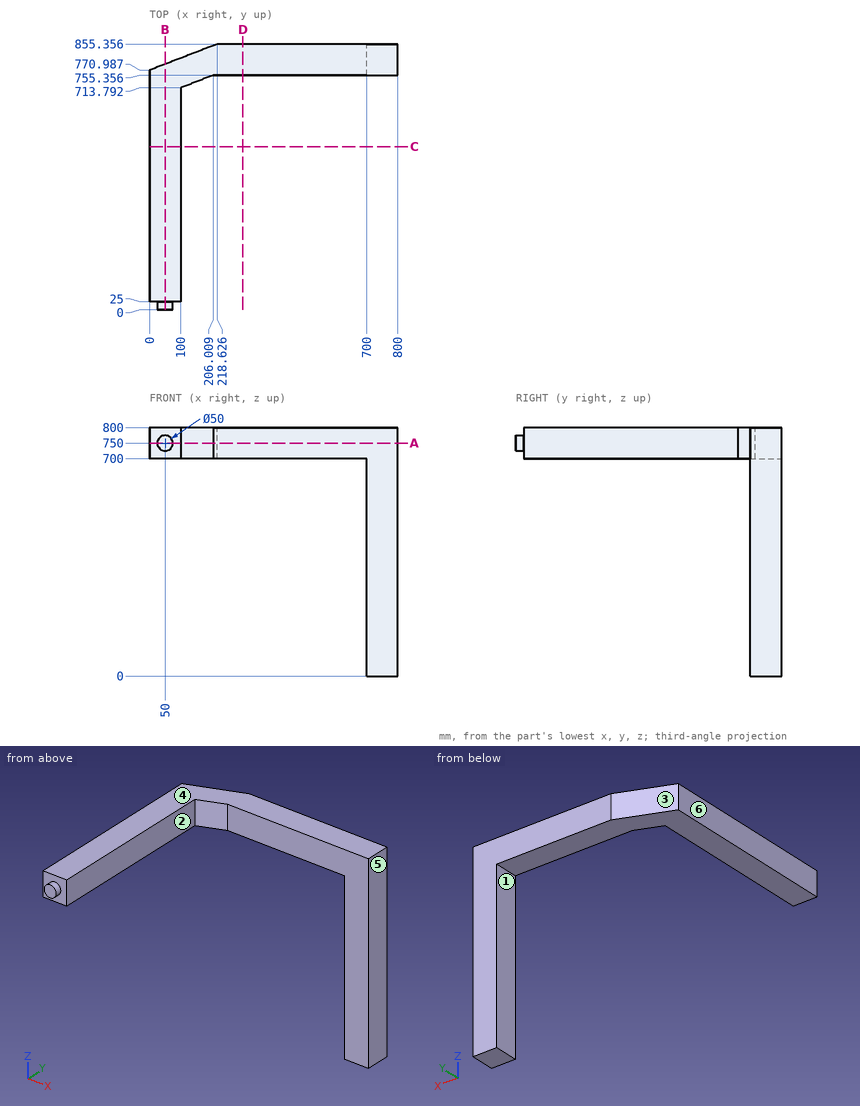
The drawing under review shows one solid part. Ordinate dimensions are in mm from its lowest x, y, z. A direction names the side the tool comes from. Round coordinates to 2 decimals unless told otherwise and drop trailing zeros. Order: outer loops, then holes, each group sorted by start corner. A loop starts at its lowest first (then second) coordinate and runs counter-clockwise, first axis right, second up. Notation, with made-up numbers: (8, 83.5) -> (28, 83.5) arc R12 cw to (28, 94.5) -> close; hole circle Ø9 at (64.25, 39.25). An arc over 180 degrees is marked (long way). Use a Markdown table: item, result.
Q1. We need section A-A on z = 750. Write out the cut boundary in (x, y) (1 decimal).
Values:
| item | result |
|---|---|
| outline | (0, 25) -> (25, 25) -> (25, 0) -> (75, 0) -> (75, 25) -> (100, 25) -> (100, 713.8) -> (206, 755.4) -> (800, 755.4) -> (800, 855.4) -> (218.6, 855.4) -> (0, 771) -> close |
Q2. We need section B-B on x = 50. Write out the cut boundary in (y, z), then the cut area to 3 significant figures.
Values:
| item | result |
|---|---|
| outline | (0, 725) -> (25, 725) -> (25, 700) -> (790.28, 700) -> (790.28, 800) -> (25, 800) -> (25, 775) -> (0, 775) -> close |
| area | 77,800 mm^2 |
Q3. We need section D-D on x = 300.5. Write out the cut boundary in (y, z), then the cut area to 3 significant figures.
Values:
| item | result |
|---|---|
| outline | (755.36, 700) -> (855.36, 700) -> (855.36, 800) -> (755.36, 800) -> close |
| area | 10,000 mm^2 |
Q4. Mouldability with a two-part tool opening along X and no side actions: class the marked faces 4, 5 and 6 as +X half, -X half, draft (parallel to the pull), parting line (faces both ways), or undercut.
Values:
| item | result |
|---|---|
| face 4 | draft |
| face 5 | +X half |
| face 6 | -X half |
Q5. We need section C-C on y = 524.5. Write out the cut boundary in (x, z), then the cut area to 3 significant figures.
Values:
| item | result |
|---|---|
| outline | (0, 700) -> (100, 700) -> (100, 800) -> (0, 800) -> close |
| area | 10,000 mm^2 |
Q6. For line 1 (X direction, y = 452, z = 735); line 2 (Z direction, x = 60.5, y = 338); line 3 (Y direction, x = 115.5, z = 747.5), list the stretches that pass through material, from the lowest coordinate up.
Values:
| item | result |
|---|---|
| line 1 | x = 0 to 100 |
| line 2 | z = 700 to 800 |
| line 3 | y = 719.87 to 815.56 |
Q7. Tool access review of the marked faces 1, 2 and 3: name each direction out of +Z, -Z, +X, -X, +Y, -Y from which nothing blocks a thin tool from reaching the whole face with its end or side.
Values:
| item | result |
|---|---|
| face 1 | -Z, -X, +Y, -Y |
| face 2 | +Z, -Z, +X, -Y |
| face 3 | +Z, -Z, -X, +Y |
